The listing builds one solid part. Answer for the finished solid, in the listing's coordinates (mm). Give positions to 0.01 mm unless a question says otherwise; leave off trailing zeros. Write each loop counter-clockwise with the first axis right and the second up, starting at its lowest first coordinate (ties: lowest second). Pieces come first, ordered by that corner, then holes. Notation, with made-up numbers: (85.25, 48) - (122.25, 48) arc R20 ccw to (122.25, 69) - close; hole circle Ø1 at (-31.5, 51.25). An arc over 180 degrees is marked (long way). One line per item, written item: value. Start each with the question number.
from build123d import *

# Parameters (mm, degrees)
F1_DEPTH = 3.175
F2_D     = 10.0838
F3_D     = 6.7564


with BuildPart() as f1:
    # F0 (on Front) → F1 (new body)
    with BuildSketch(Plane.XZ):
        with BuildLine():
            Line((-4.9834776765, 44.439300983), (-58.7851488975, 11.408687969))
            ThreePointArc((-58.7851488975, 11.408687969), (-61.490054873, 4.4851244515), (-55.5625, 0))
            Line((-55.5625, 0), (0, 0))
            Line((0, 0), (55.5625, 0))
            ThreePointArc((55.5625, 0), (61.490054873, 4.4851244515), (58.7851488975, 11.408687969))
            Line((58.7851488975, 11.408687969), (4.9834776765, 44.439300983))
            ThreePointArc((4.9834776765, 44.439300983), (2.589240539, 45.4883219686), (0, 45.847))
            ThreePointArc((0, 45.847), (-2.589240539, 45.4883219686), (-4.9834776765, 44.439300983))
        make_face()
    extrude(amount=F1_DEPTH)

    # F2 (through all)
    with Locations(Plane(origin=(0, 0, 0), x_dir=(1, 0, 0), z_dir=(0, 1, 0))):
        with Locations((0, -36.322)):
            Hole(F2_D / 2)

    # F3 (through all)
    with Locations(Plane(origin=(0, 0, 0), x_dir=(1, 0, 0), z_dir=(0, 1, 0))):
        with Locations((55.5625, -6.1595), (-55.5625, -6.1595)):
            Hole(F3_D / 2)


solid = f1.part
Item 1: Each of these flat-tipped pins is pushed along its axis until it touches: pin 1 Ø1.5 at (x, y) = (-25.5, -0.5) entering from +Z; pin 2 Ø9 at (x, z) = (0, 36.322) entering from -Y. Where does it stop, or does it pass through?
Item 2: Find section B-B on y = -1. Give the number of separate pieces and of enclosed holes in the cut face, plus the area to 3 significant figures.
Item 3: Find section C-C on x = -27. Determine the outline of the cut face in (y, z) (3 decimals), plus the area to 3 significant figures.
Item 4: Straight lines are drawn through the part: line 1 along X through (y, z) = (-0.6, 8.5); line 2 along Z through (x, y) = (0, -2.4); line 3 along X through (y, z) = (-1.8, 38.5). For each, find the intervals that lie inside material, in ascending order.
Item 5: The mould has two halves that part along Z. Classify faces 1 (the cylindrical face through (-61.52, -1.57, 4.59)), 2 (the flat face through (-31.508, -1.565, 28.155)), 3 (the cylindrical face through (1.093, -1.61, 41.244)): +Z half, -Z half, draft (parallel to the pull), parting line (faces both ways), or undercut.
Item 6: Find section A-A on z = 5. Determine the outline of the cut face in (x, y) (3 decimals).
Item 7: Find section D-D on x = -50. Determine the outline of the cut face in (y, z) (3 decimals).
Values:
1. pin 1: z = 32.3
1. pin 2: through
2. separate pieces: 1
2. enclosed holes: 3
2. area: 3,350 mm^2
3. outline: (-3.175, 0) - (0, 0) - (0, 30.923) - (-3.175, 30.923) - close
3. area: 98.2 mm^2
4. line 1: -61.26 to -58, -53.13 to 53.13, 58 to 61.26
4. line 2: 0 to 31.28, 41.36 to 45.85
4. line 3: -14.66 to -4.55, 4.55 to 14.66
5. face 1: parting line
5. face 2: +Z half
5. face 3: undercut
6. outline: (-61.612, -3.175) - (-58.735, -3.175) - (-58.735, 0) - (-61.612, 0) - close; (-52.39, -3.175) - (52.39, -3.175) - (52.39, 0) - (-52.39, 0) - close; (58.735, -3.175) - (61.612, -3.175) - (61.612, 0) - (58.735, 0) - close
7. outline: (-3.175, 0) - (0, 0) - (0, 16.802) - (-3.175, 16.802) - close
